Can you work these out from the drawing? Everything is in mm from the part's minimum corner. A direction names the side the tool comes from. Coordinates: 2 decimals unless noted, no trailing zeros. Write each loop counter-clockwise with the first axis right and the second up, starting at its lowest first coordinate (ties: lowest second). Pieces come first, ordered by that corner, then holes. Notation, with made-up numbers: M -29.5,38 L 4.5,38 A10 ccw 4.5,44 Z; hole C 17,16 d1. An arc over 180 degrees is marked long. Write each question's results on one line, items separated by ' | '. Start each with the question number.
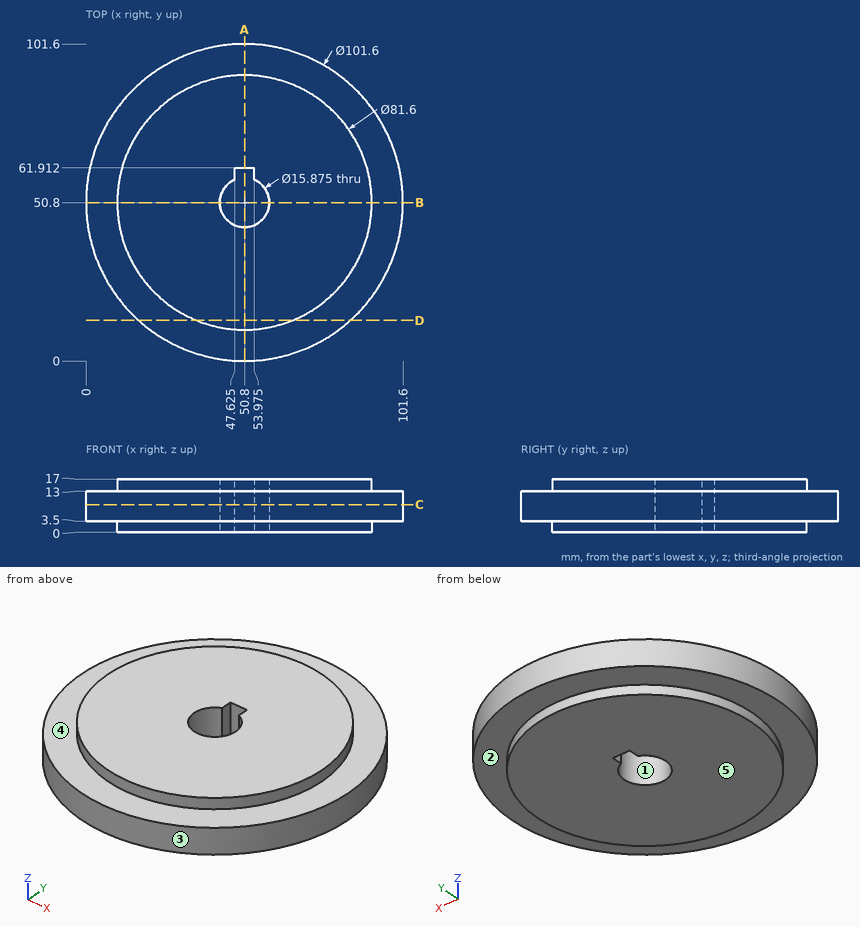
1) I want a section at B-B, the plane y = 50.8. Write out the boundary of the cut face in (x, z).
2) I want a section at A-A, the plane x = 50.8. Write out the boundary of the cut face in (y, z).
3) For pin 1 Ø4 at (y, z) = (60.5, 8) entering from -X; pin 2 Ø4 at (y, z) = (41, 2.5) entering from -X (1 decimal); pin 3 Ø5 at (x, z) = (21.5, 14.5) entering from -Y, each with a flat end and sliding along its axis, tell me the tip position at first contact or that it passes through.
4) I want a section at D-D, the plane y = 13. Write out the boundary of the cut face in (x, z) (1 decimal), then the cut area to 3 significant figures.
5) We'd pull the mould along Y, two halves only. Please class the marked faces 1, 2 and 3: pulls with the +Y half, pulls with the -Y half, needs draft (parallel to the pull), parting line crosses it, or undercut.
6) Please list where these lines run through material, in increasing order: line 1 (Y direction, x = 50.8, z = 8.5); line 2 (Z direction, x = 52.5, y = 97.5); line 3 (Y direction, x = 52.5, z = 5). Write a range as [from, to].
7) I want a section at C-C, the plane z = 8.75. Write out the boundary of the cut face in (x, y) (1 decimal).
8) For the marked faces 4 and 5, which set-ups out of +Z, -Z, +X, -X, +Y, -Y let a thin tool reach every point of the face, with its end or its side?
Output:
1) outline: M 0,3.5 L 10,3.5 L 10,0 L 42.86,0 L 42.86,17 L 10,17 L 10,13 L 0,13 Z; M 58.74,0 L 91.6,0 L 91.6,3.5 L 101.6,3.5 L 101.6,13 L 91.6,13 L 91.6,17 L 58.74,17 Z
2) outline: M 0,3.5 L 10,3.5 L 10,0 L 42.86,0 L 42.86,17 L 10,17 L 10,13 L 0,13 Z; M 61.91,0 L 91.6,0 L 91.6,3.5 L 101.6,3.5 L 101.6,13 L 91.6,13 L 91.6,17 L 61.91,17 Z
3) pin 1: stops at x = 0.59 | pin 2: stops at x = 0.6 | pin 3: stops at y = 7.96
4) outline: M 16.9,3.5 L 35.4,3.5 L 35.4,0 L 66.2,0 L 66.2,3.5 L 84.7,3.5 L 84.7,13 L 66.2,13 L 66.2,17 L 35.4,17 L 35.4,13 L 16.9,13 Z | area: 875 mm2
5) face 1: undercut | face 2: needs draft | face 3: parting line crosses it
6) line 1: y = [0, 42.86], [61.91, 101.6] | line 2: z = [3.5, 13] | line 3: y = [0.03, 43.05], [61.91, 101.57]
7) outline: C 50.8,50.8 d101.6; hole M 47.6,58.1 A7.9 ccw long 54,58.1 L 54,61.9 L 47.6,61.9 Z
8) face 4: +Z | face 5: -Z, +X, -X, +Y, -Y
